For this review, use the dimensioned drawing (mm, ordinates from the lowest corner) and the shaded views. A direction names the side the tool comes from. Round coordinates to 2 decimals unless told otherwise and drop trailing zeros. Loops run counter-clockwise (first coordinate to the right, second up) from the corner with the lowest first, then second, coordinate; pieces in that order, holes last. Notation, with made-up numbers: (70.5, 16) - (100.5, 16) arc R32 cw to (100.5, 44) - close; hole circle Ø3 at (29, 51). An arc over 180 degrees is marked (long way). Return JSON: item names as keys, results as strings. Group by question number.
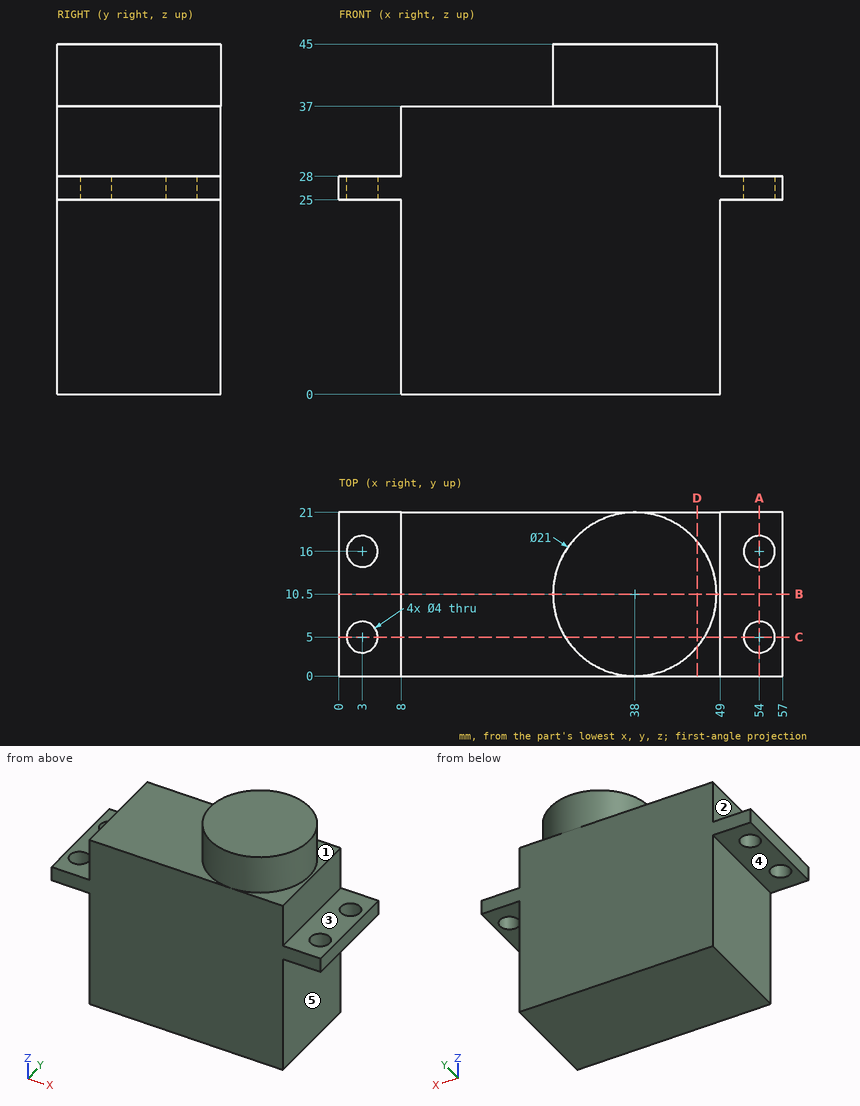
Q1. Add section A-A, the plane x = 54. State the section outline as (y, z) points.
Q2. Insertion check: pin 1 Ø4.5 at (y, z) = (8, 33) entering from +X; pin 2 Ø6.5 at (x, y) = (3, 5) entering from -Z; pin 3 Ø8 at (y, z) = (12.5, 38.5) entering from -X; pin 4 Ø3 at (x, y) = (54, 16) entering from +Z. Each pin has a flat end and moves straight along its axis. Give the tip position at first contact, or say it passes through.
Q3. Add section D-D, the plane x = 46. State the section outline as (y, z) points, plus the area to 3 significant figures.
Q4. For line 1 (Y direction, x = 54, z = 26); line 2 (Z direction, x = 50, y = 1.5); line 3 (Z direction, x = 27, y = 9.5), list the stretches that pass through material, from the lowest coordinate up.
Q5. Add section B-B, the plane y = 10.5. State the section outline as (x, z) points.
Q6. Tool access review of the marked faces 1, 2, 3, 4 and 5: name each direction out of +Z, -Z, +X, -X, +Y, -Y from which nothing blocks a thin tool from reaching the whole face with its end or side.
Q7. Add section C-C, the plane y = 5. State the section outline as (x, z) points, plus the area to 3 significant figures.
Evaluation:
{
 "1": {"outline": "(0, 25) - (3, 25) - (3, 28) - (0, 28) - close; (7, 25) - (14, 25) - (14, 28) - (7, 28) - close; (18, 25) - (21, 25) - (21, 28) - (18, 28) - close"},
 "2": {"pin 1": "x = 49", "pin 2": "z = 25", "pin 3": "x = 8", "pin 4": "through"},
 "3": {"outline": "(0, 0) - (21, 0) - (21, 37) - (17.3, 37) - (17.3, 45) - (3.7, 45) - (3.7, 37) - (0, 37) - close", "area": "886 mm²"},
 "4": {"line 1": "0 to 3, 7 to 14, 18 to 21", "line 2": "25 to 28", "line 3": "0 to 37"},
 "5": {"outline": "(0, 25) - (8, 25) - (8, 0) - (49, 0) - (49, 25) - (57, 25) - (57, 28) - (49, 28) - (49, 37) - (48.5, 37) - (48.5, 45) - (27.5, 45) - (27.5, 37) - (8, 37) - (8, 28) - (0, 28) - close"},
 "6": {"face 1": "+Z, +X", "face 2": "+Z, -X, +Y, -Y", "face 3": "+Z, +X, +Y, -Y", "face 4": "-Z, -X, +Y, -Y", "face 5": "-Z, +X, +Y, -Y"},
 "7": {"outline": "(0, 25) - (1, 25) - (1, 28) - (0, 28) - close; (5, 25) - (8, 25) - (8, 0) - (49, 0) - (49, 25) - (52, 25) - (52, 28) - (49, 28) - (49, 37) - (46.94, 37) - (46.94, 45) - (29.06, 45) - (29.06, 37) - (8, 37) - (8, 28) - (5, 28) - close; (56, 25) - (57, 25) - (57, 28) - (56, 28) - close", "area": "1,680 mm²"}
}
